For this review, take the finished solid that the model builds, in its own axes (mm). Face numbers are marked on the shaded views. A direction names the side the tool comes from. Give positions to 0.01 mm unless a question says otherwise; leave off trailing zeros. Loops run counter-clockwise (first coordinate to the right, second up) from the corner with the lowest first, then second, coordinate; pieces in that order, holes last. Notation, with made-up numbers: (74, -25) - (105, -25) arc R25 cw to (105, -11) - close; hole circle Ø2 at (19.5, 3.25). An arc over 180 degrees is marked (long way). Use CSV: the item, a comma, the result in double quotes. Start each with the question number.
1. For pin 1 (21 mm diameter, centred on y = 6, z = -15.5, fed in from -X); pin 2 (1.6 mm diameter, centred on x = -35, z = -43.5, fed in from -Y); pin 3 (6.5 mm diameter, centred on x = 0, z = 0, fed in from -Y); pin 4 (4 mm diameter, centred on x = 24, y = -18, fed in from -Z), all flat-tipped, find the tip position at first contact; note any pin that passes through.
2. Take a section at C-C on x = 28. Give the boundary of the cut face in (y, z).
3. Mouldability with a two-part tool opening along X and no side actions: class the marked faces 5, 6 and 7 as pulls with the +X half, pulls with the -X half, needs draft (parallel to the pull), parting line crosses it, or undercut.
4. Take a section at B-B on y = -8. Give the boundary of the cut face in (x, z), plus the area to 3 significant figures.
5. Take a section at D-D on z = 30.5. Give the boundary of the cut face in (x, y), plus the area to 3 significant figures.
6. For the marked faces 1, 2, 3 and 4, list the 3-axis set-ups (+Z, -Z, +X, -X, +Y, -Y) from which the entire face can be reached by the end or side of a thin tool; tool diameter is ignored.
7. Take a section at A-A on y = 0. State how many separate pieces and enclosed holes the cut face has, plus the area to 3 significant figures.
8. Wall thickness on line 1 (X direction, y = -3, z = 0); line 2 (Y direction, x = -37, z = -20); line 3 (X direction, y = -24.5, z = -5): over which ranges is each line inside the solid? List them lowest first.
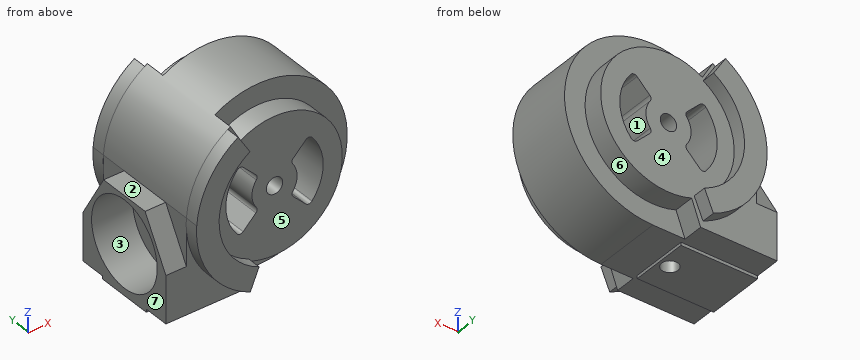
```python
from build123d import *

# Parameters (mm, degrees)
SKETCH1_R           = 4
BOSS_EXTRUDE1_DEPTH = 26.56
CUT_EXTRUDE1_START  = -10
CUT_EXTRUDE1_DEPTH  = 10
BOSS_EXTRUDE2_DEPTH = 6.6
CUT_EXTRUDE2_DEPTH  = 10
SKETCH4_R           = 21
CUT_EXTRUDE3_DEPTH  = 20
SKETCH5_W           = 37.244501106
SKETCH5_H           = 28
BOSS_EXTRUDE3_DEPTH = 1.5
SKETCH7_R           = 4


with BuildPart() as part:
    # Sketch1 → Boss-Extrude1 (new body)
    with BuildSketch(Plane(origin=(0, 0, 0), x_dir=(1, 0, 0), z_dir=(0, 1, 0))):
        with BuildLine():
            Line((0, 43), (-52.895221179, 43))
            Line((-52.895221179, 43), (-52.895221179, -3))
            Line((-52.895221179, -3), (-42.895221179, -3))
            ThreePointArc((-42.895221179, -3), (31.448370387, -29.325756597), (0, 43))
        make_face()
        with Locations(Location((0, 0, 0), (0, 0, 90))):
            Circle(SKETCH1_R, mode=Mode.SUBTRACT)
        with BuildLine():
            Line((-15.278907029, -15.278907029), (-9.082951062, -9.082951062))
            ThreePointArc((-9.082951062, -9.082951062), (-8.503126103, -7.8230436), (-8.882216221, -6.488931731))
            ThreePointArc((-8.882216221, -6.488931731), (-11, 0), (-8.882216221, 6.488931731))
            ThreePointArc((-8.882216221, 6.488931731), (-8.503126103, 7.8230436), (-9.082951062, 9.082951062))
            Line((-9.082951062, 9.082951062), (-15.278907029, 15.278907029))
            ThreePointArc((-15.278907029, 15.278907029), (-16.785384719, 15.862564166), (-18.231657051, 15.142545399))
            ThreePointArc((-18.231657051, 15.142545399), (-23.7, 0), (-18.231657051, -15.142545399))
            ThreePointArc((-18.231657051, -15.142545399), (-16.785384719, -15.862564166), (-15.278907029, -15.278907029))
        make_face(mode=Mode.SUBTRACT)
        with BuildLine():
            Line((15.278907029, 15.278907029), (9.082951062, 9.082951062))
            ThreePointArc((9.082951062, 9.082951062), (8.503126103, 7.8230436), (8.882216221, 6.488931731))
            ThreePointArc((8.882216221, 6.488931731), (11, 0), (8.882216221, -6.488931731))
            ThreePointArc((8.882216221, -6.488931731), (8.503126103, -7.8230436), (9.082951062, -9.082951062))
            Line((9.082951062, -9.082951062), (15.278907029, -15.278907029))
            ThreePointArc((15.278907029, -15.278907029), (16.785384719, -15.862564166), (18.231657051, -15.142545399))
            ThreePointArc((18.231657051, -15.142545399), (23.7, 0), (18.231657051, 15.142545399))
            ThreePointArc((18.231657051, 15.142545399), (16.785384719, 15.862564166), (15.278907029, 15.278907029))
        make_face(mode=Mode.SUBTRACT)
    boss_extrude1 = extrude(amount=BOSS_EXTRUDE1_DEPTH)

    # Sketch2 → Cut-Extrude1 (cut)
    with BuildSketch(Plane(origin=(0, 26.56, 0), x_dir=(1, 0, 0), z_dir=(0, 1, 0)).offset(CUT_EXTRUDE1_START)):
        with BuildLine():
            Line((-16.5, -28.578838325), (-21.5, -37.239092363))
            ThreePointArc((-21.5, -37.239092363), (41.53481053, -11.129218939), (0, 43))
            Line((0, 43), (-15.650720073, 43))
            Line((-15.650720073, 43), (-11.28666473, 31.009856486))
            ThreePointArc((-11.28666473, 31.009856486), (32.874425037, -2.876139511), (-16.5, -28.578838325))
        make_face()
    cut_extrude1 = extrude(amount=CUT_EXTRUDE1_DEPTH, mode=Mode.SUBTRACT)

    # Sketch2<3> → Boss-Extrude2 (add)
    with BuildSketch(Plane(origin=(0, 26.56, 0), x_dir=(1, 0, 0), z_dir=(0, 1, 0))):
        with BuildLine():
            ThreePointArc((-42.895221179, -3), (-36.85807218, -22.146839847), (-22.786528362, -36.466068135))
            Line((-22.786528362, -36.466068135), (-16.957416455, -27.137539077))
            ThreePointArc((-16.957416455, -27.137539077), (-31.902604506, 2.494759659), (-12.532809858, 29.443652577))
            Line((-12.532809858, 29.443652577), (-16.840963246, 39.56490815))
            ThreePointArc((-16.840963246, 39.56490815), (-36.674865833, 22.448924609), (-42.895221179, -3))
        make_face()
    boss_extrude2 = extrude(amount=BOSS_EXTRUDE2_DEPTH)

    # Mirror1: Boss-Extrude1, Cut-Extrude1, Boss-Extrude2 across plane
    add(boss_extrude1.mirror(Plane.ZX))
    add(cut_extrude1.mirror(Plane.ZX), mode=Mode.SUBTRACT)
    add(boss_extrude2.mirror(Plane.ZX))

    # Sketch3 → Cut-Extrude2 (cut)
    with BuildSketch(Plane.ZY.offset(52.895221179)):
        Polygon((-19.982907976, 26.548244298), (3, 13.279056191), (3, 26.56), (-20.003269449, 26.56), (-20, 26.558112383), align=None)
        Polygon((3, -26.56), (3, -13.279056191), (-20, -26.558112383), (-20.003269449, -26.56), align=None)
    extrude(amount=-CUT_EXTRUDE2_DEPTH, mode=Mode.SUBTRACT)

    # Sketch4 → Cut-Extrude3 (cut)
    with BuildSketch(Plane.ZY.offset(52.895221179)):
        with Locations((-20, 0)):
            Circle(SKETCH4_R)
    extrude(amount=-CUT_EXTRUDE3_DEPTH, mode=Mode.SUBTRACT)

    # Sketch5 → Boss-Extrude3 (add)
    with BuildSketch(Plane(origin=(0, 0, -43), x_dir=(-1, 0, 0), z_dir=(0, 0, -1))):
        with Locations((34.272970626, 0)):
            Rectangle(SKETCH5_W, SKETCH5_H)
    extrude(amount=BOSS_EXTRUDE3_DEPTH)

    # Cut-Sweep3: sweep along a path in Sketch6
    with BuildLine(Plane(origin=(0, 0, 0), x_dir=(1, 0, 0), z_dir=(0, 1, 0))) as cut_sweep3_path:
        Line((-52.895221179, 20), (-32.895221179, 20))
        ThreePointArc((-32.895221179, 20), (-24.409939805, 23.514718626), (-20.895221179, 32))
        Line((-20.895221179, 32), (-20.895221179, 44.5))
    # Sketch7 → Cut-Sweep3 (sweep, cut)
    with BuildSketch(Plane(origin=(0, 0, -44.5), x_dir=(-1, 0, 0), z_dir=(0, 0, -1))):
        with Locations((20.895221179, 0)):
            Circle(SKETCH7_R)
    sweep(path=cut_sweep3_path.line, mode=Mode.SUBTRACT)


solid = part.part
```
Check result:
1,pin 1,"stops at x = -32.9"
1,pin 2,"stops at y = -26.56"
1,pin 3,"passes through"
1,pin 4,"stops at z = -36.57"
2,outline,"(-26.56, -17.46) - (-16.56, -17.46) - (-16.56, -32.63) - (16.56, -32.63) - (16.56, -17.46) - (26.56, -17.46) - (26.56, 17.46) - (16.56, 17.46) - (16.56, 32.63) - (-16.56, 32.63) - (-16.56, 17.46) - (-26.56, 17.46) - close"
3,face 5,"needs draft"
3,face 6,"undercut"
3,face 7,"pulls with the -X half"
4,outline,"(-52.9, -44.5) - (-15.65, -44.5) - (-15.65, -43) - (0, -43) arc R43 ccw (long way) to (-42.9, 3) - (-52.9, 3) - (-52.9, -0.58) - (-32.9, -0.58) - (-32.9, -39.42) - (-52.9, -39.42) - close; hole (-18.23, -15.14) arc R2 ccw to (-15.28, -15.28) - (-9.08, -9.08) arc R2 ccw to (-8.88, -6.49) arc R11 cw to (-8.88, 6.49) arc R2 ccw to (-9.08, 9.08) - (-15.28, 15.28) arc R2 ccw to (-18.23, 15.14) arc R23.7 ccw to start; hole circle Ø8 at (0, 0); hole (8.88, -6.49) arc R2 ccw to (9.08, -9.08) - (15.28, -15.28) arc R2 ccw to (18.23, -15.14) arc R23.7 ccw to (18.23, 15.14) arc R2 ccw to (15.28, 15.28) - (9.08, 9.08) arc R2 ccw to (8.88, 6.49) arc R11 cw to start"
4,area,"5,200 mm²"
5,outline,"(-30.31, -33.16) - (-19.06, -33.16) - (-19.06, -26.56) - (-17.61, -26.56) - (-17.61, -16.56) - (-12.6, -16.56) - (-12.6, -26.56) - (12.6, -26.56) - (12.6, -16.56) - (30.31, -16.56) - (30.31, 16.56) - (12.6, 16.56) - (12.6, 26.56) - (-12.6, 26.56) - (-12.6, 16.56) - (-17.61, 16.56) - (-17.61, 26.56) - (-19.06, 26.56) - (-19.06, 33.16) - (-30.31, 33.16) - close"
5,area,"2,910 mm²"
6,face 1,"+Y, -Y"
6,face 2,"+Z, -X, +Y, -Y"
6,face 3,"-X"
6,face 4,"+Y"
7,separate pieces,"2"
7,enclosed holes,"3"
7,area,"4,890 mm²"
8,line 1,"x = -32.9 to -23.7, -11 to -4, 4 to 11, 23.7 to 43"
8,line 2,"y = -33.16 to -21, 21 to 33.16"
8,line 3,"x = -42.9 to -23.17, -9.8 to 9.8, 23.17 to 32.62"
